CAD build for the part. Positions are in the model's coordinates, mm. A direction names the side the tool comes from. Coordinates: 2 decimals unless noted, no trailing zeros. Loops run counter-clockwise (first coordinate to the right, second up) from the corner with the lowest first, then second, coordinate; pieces in that order, holes last. Notation, with made-up numbers: (34, 88.25) -> (52, 88.25) arc R17 cw to (52, 112.25) -> close; hole circle Ø2 at (34, 56.5). An arc over 180 degrees is marked (long way). Write each question's results on one line, items separated by ' | '.
from build123d import *

# Parameters (mm, degrees)
BOSS_EXTRUDE1_DEPTH = 254
BOSS_EXTRUDE2_DEPTH = 762
BOSS_EXTRUDE3_DEPTH = 1016


with BuildPart() as part:
    # Sketch1 → Boss-Extrude1 (new body)
    with BuildSketch(Plane(origin=(0, 0, 0), x_dir=(1, 0, 0), z_dir=(0, 1, 0))):
        Polygon((762, 508), (508, 508), (254, -508), (1016, -508), align=None)
    extrude(amount=BOSS_EXTRUDE1_DEPTH)

    # Sketch1<3> → Boss-Extrude2 (add)
    with BuildSketch(Plane(origin=(0, 0, 0), x_dir=(1, 0, 0), z_dir=(0, 1, 0))):
        Polygon((508, 508), (254, 508), (0, -508), (254, -508), align=None)
    extrude(amount=BOSS_EXTRUDE2_DEPTH)

    # Sketch1<4> → Boss-Extrude3 (add)
    with BuildSketch(Plane(origin=(0, 0, 0), x_dir=(1, 0, 0), z_dir=(0, 1, 0))):
        with BuildLine():
            Line((254, 508), (0, 508))
            ThreePointArc((0, 508), (-508, 0), (0, -508))
            Line((0, -508), (254, 508))
        make_face()
    extrude(amount=BOSS_EXTRUDE3_DEPTH)


solid = part.part
1) Pin check, flat tips, straight feed: pin 1 (2 mm diameter, centred on y = 482, z = -85.5, fed in from -X); pin 2 (5 mm diameter, centred on x = -355, y = 173.5, fed in from -Z); pin 3 (5 mm diameter, centred on y = 854, z = -226.5, fed in from +X). Stop position of each tip, or through.
Outcome:
pin 1: stops at x = -500.92 | pin 2: stops at z = -365.8 | pin 3: stops at x = 184.25
2) Slice it at D-D (x = 362.5). Write the cut outline in (y, z).
Outcome:
outline: (0, -508) -> (762, -508) -> (762, 74) -> (254, 74) -> (254, 508) -> (0, 508) -> close
3) Which spindle directions (+Z, -Z, +X, -X, +Y, -Y) get a long thin tool onto all of the face, cutting with end or side? Do faces 1 (the flat face through (302, 388, -508)), 2 (the flat face through (250, 762, -7)). Say none if no direction does.
Outcome:
face 1: -Z, +X, -X, +Y, -Y | face 2: +Z, +X, +Y
4) Slice it at A-A (z = 0). Write the cut outline in (x, y).
Outcome:
outline: (-508, 0) -> (889, 0) -> (889, 254) -> (381, 254) -> (381, 762) -> (127, 762) -> (127, 1016) -> (-508, 1016) -> close
5) Slice it at C-C (y = 422). Write the cut outline in (x, z), then the cut area to 3 significant figures.
Outcome:
outline: (0, -508) -> (508, -508) -> (254, 508) -> (0, 508) arc R508 ccw to start | area: 792,000 mm^2
6) Drill centre lines: L1, parallel to Y at x = 615.5, z = 74; L2, parallel to Y at x = 243, z = 150; L3, parallel to X at y = 74, z = -245. Where is each one in solid material? Low to high. Write a range as from..to.
Outcome:
L1: y = 0..254 | L2: y = 0..762 | L3: x = -445.02..827.75
7) Slice it at B-B (x = 89). Write the cut outline in (y, z), then the cut area to 3 significant figures.
Outcome:
outline: (0, -508) -> (1016, -508) -> (1016, 152) -> (762, 152) -> (762, 508) -> (0, 508) -> close | area: 942,000 mm^2
